Build history of the part. All positions in model axes, mm. A direction names the side the tool comes from. Give positions to 0.01 mm unless a question says otherwise; leave off trailing zeros. Return JSON: item names as keys, results as strings. Group by question number.
1) 3-axis set-ups, long thin cutter, end or side, ignore diameter. For faces 1 (the face through (96.99, 2.85, 17.74)), 2 (the face through (39.646, 2, 16)): which of +Z, -Z, +X, -X, +Y, -Y reach the whole face in a straight line?
2) Drill centre lines: probe 1 along Y at (x, z) = (92.5, 24); probe 2 along Y at (x, z) = (91.5, 24). Where is each one in solid material? Low to high. Write a range as from..to.
3) Mould opens along Z. For faces 3 (the face through (60, 5, 16)), 4 (the face through (100, 49, 17)), 5 (the face through (49, 51, 35)) say: released by +Z, released by -Z, zero draft, split by the parting line, or undercut.
4) Drop flat-ended pins along their axis: pin 1 (1.5 mm diameter, centred on y = 2, z = 16, fed in from -X); pin 2 (3.5 mm diameter, centred on y = 2, z = 17, fed in from +X); pin 3 (1.3 mm diameter, centred on x = 46.5, z = 15, fed in from -Y). Give the stop position or say it passes through.
```python
from build123d import *

# Parameters (mm, degrees)
SKETCH1_W           = 100
SKETCH1_H           = 100
BOSS_EXTRUDE1_DEPTH = 35
FILLET1_R           = 10
SKETCH2_W           = 9.403715906
SKETCH2_H           = 4.36940335
SKETCH2_W_2         = 10.971001891
SKETCH2_H_2         = 8.786300215
SKETCH2_W_3         = 11.255962979
SKETCH2_H_3         = 3.087078454
SKETCH2_W_4         = 10.021131597
SKETCH2_H_4         = 3.03958494
CUT_EXTRUDE1_DEPTH  = 5


with BuildPart() as part:
    # Sketch1 → Boss-Extrude1 (new body)
    with BuildSketch(Plane.XY):
        with Locations((50, 50)):
            Rectangle(SKETCH1_W, SKETCH1_H)
    extrude(amount=BOSS_EXTRUDE1_DEPTH)

    # Fillet1
    fillet1_edges = [part.edges().sort_by_distance(p)[0] for p in [
        (0, 100, 17.5),
        (100, 100, 17.5),
        (100, 0, 17.5),
        (0, 0, 17.5),
    ]]
    fillet(fillet1_edges, radius=FILLET1_R)

    # Sketch2 → Cut-Extrude1 (cut)
    with BuildSketch(Plane.XZ):
        with Locations((44.348271753, 16.241421861)):
            Rectangle(SKETCH2_W, SKETCH2_H)
        with Locations((24.709703434, 18.544857323)):
            Rectangle(SKETCH2_W_2, SKETCH2_H_2)
        with Locations((74.672880875, 15.885220501)):
            Rectangle(SKETCH2_W_3, SKETCH2_H_3)
        with Locations((60.377332957, 15.671499685)):
            Rectangle(SKETCH2_W_4, SKETCH2_H_4)
    extrude(amount=-CUT_EXTRUDE1_DEPTH, mode=Mode.SUBTRACT)


solid = part.part
```
Results:
{
 "1": {"face 1": "+Z, -Z, +X, -Y", "face 2": "-Y"},
 "2": {"probe 1": "0.32..99.68", "probe 2": "0.11..99.89"},
 "3": {"face 3": "undercut", "face 4": "zero draft", "face 5": "released by +Z"},
 "4": {"pin 1": "x = 3.11", "pin 2": "x = 97.81", "pin 3": "y = 5"}
}
